```python
from build123d import *

# Parameters (mm, degrees)
MODEL_R             = 1.4605
MODEL_R_2           = 2
BOSS_EXTRUDE1_DEPTH = 2.413
SKETCH1_W           = 10
SKETCH1_H           = 24
CUT_EXTRUDE1_DEPTH  = 10


with BuildPart() as part:
    # Model → Boss-Extrude1 (new body, symmetric)
    with BuildSketch(Plane.XY):
        with BuildLine():
            Line((-290.681304326, -31.2683), (-258.931304326, -12.937428953))
            Line((-258.931304326, -12.937428953), (-258.931304326, -5.149171047))
            Line((-258.931304326, -5.149171047), (-290.681304326, 13.1817))
            Line((-290.681304326, 13.1817), (-290.681304326, 51.2817))
            Line((-290.681304326, 51.2817), (-258.931304326, 69.612571047))
            Line((-258.931304326, 69.612571047), (-258.931304326, 76.6817))
            Line((-258.931304326, 76.6817), (-290.681304326, 108.4317))
            Line((-290.681304326, 108.4317), (-290.681304326, 127.4817))
            ThreePointArc((-290.681304326, 127.4817), (-288.821432386, 131.971828061), (-284.331304326, 133.8317))
            Line((-284.331304326, 133.8317), (-265.281304326, 133.8317))
            Line((-265.281304326, 133.8317), (-227.181304326, 95.7317))
            Line((-227.181304326, 95.7317), (-23.981304326, 95.7317))
            Line((-23.981304326, 95.7317), (14.118695674, 133.8317))
            Line((14.118695674, 133.8317), (33.168695674, 133.8317))
            ThreePointArc((33.168695674, 133.8317), (37.658823735, 131.971828061), (39.518695674, 127.4817))
            Line((39.518695674, 127.4817), (39.518695674, 108.4317))
            Line((39.518695674, 108.4317), (7.768695674, 76.6817))
            Line((7.768695674, 76.6817), (7.768695674, 69.612571047))
            Line((7.768695674, 69.612571047), (39.518695674, 51.2817))
            Line((39.518695674, 51.2817), (39.518695674, 13.1817))
            Line((39.518695674, 13.1817), (7.768695674, -5.149171047))
            Line((7.768695674, -5.149171047), (7.768695674, -12.937428953))
            Line((7.768695674, -12.937428953), (39.518695674, -31.2683))
            Line((39.518695674, -31.2683), (39.518695674, -59.836710662))
            Line((39.518695674, -59.836710662), (10.464640386, -80.18057919))
            Line((10.464640386, -80.18057919), (7.768695674, -82.0683))
            Line((7.768695674, -82.0683), (7.768695674, -139.2183))
            Line((7.768695674, -139.2183), (39.518695674, -170.9683))
            Line((39.518695674, -170.9683), (39.518695674, -190.0183))
            ThreePointArc((39.518695674, -190.0183), (37.658823735, -194.508428061), (33.168695674, -196.3683))
            Line((33.168695674, -196.3683), (14.118695674, -196.3683))
            Line((14.118695674, -196.3683), (-23.981304326, -158.2683))
            Line((-23.981304326, -158.2683), (-227.181304326, -158.2683))
            Line((-227.181304326, -158.2683), (-265.281304326, -196.3683))
            Line((-265.281304326, -196.3683), (-284.331304326, -196.3683))
            ThreePointArc((-284.331304326, -196.3683), (-288.821432386, -194.508428061), (-290.681304326, -190.0183))
            Line((-290.681304326, -190.0183), (-290.681304326, -170.9683))
            Line((-290.681304326, -170.9683), (-258.931304326, -139.2183))
            Line((-258.931304326, -139.2183), (-258.931304326, -82.0683))
            Line((-258.931304326, -82.0683), (-290.681304326, -50.3183))
            Line((-290.681304326, -50.3183), (-290.681304326, -31.2683))
        make_face()
        with Locations((-287.125304326, -190.6025)):
            Circle(MODEL_R, mode=Mode.SUBTRACT)
        with Locations((33.752895674, -190.6025)):
            Circle(MODEL_R, mode=Mode.SUBTRACT)
        with Locations((33.752895674, 130.2757)):
            Circle(MODEL_R, mode=Mode.SUBTRACT)
        with Locations((-287.125304326, 130.2757)):
            Circle(MODEL_R, mode=Mode.SUBTRACT)
        with Locations((-274.681304256, -45.4288)):
            Circle(MODEL_R, mode=Mode.SUBTRACT)
        with Locations((-254.681304256, -45.4288)):
            Circle(MODEL_R, mode=Mode.SUBTRACT)
        with Locations((23.518695604, -45.4288)):
            Circle(MODEL_R, mode=Mode.SUBTRACT)
        with Locations((3.518695604, -45.4288)):
            Circle(MODEL_R, mode=Mode.SUBTRACT)
        with Locations((23.518695604, 30.5682)):
            Circle(MODEL_R, mode=Mode.SUBTRACT)
        with Locations((3.518695604, 30.5682)):
            Circle(MODEL_R, mode=Mode.SUBTRACT)
        with Locations((-254.681304256, 30.5682)):
            Circle(MODEL_R, mode=Mode.SUBTRACT)
        with Locations((-274.681304256, 30.5682)):
            Circle(MODEL_R, mode=Mode.SUBTRACT)
        with Locations((-125.581304326, -12.2183)):
            Circle(MODEL_R_2, mode=Mode.SUBTRACT)
        with Locations((-125.581304326, -50.3183)):
            Circle(MODEL_R_2, mode=Mode.SUBTRACT)
        Polygon((-30.331304326, -145.5683), (-68.431304326, -107.4683), (-182.731304326, -107.4683), (-220.831304326, -145.5683), align=None, mode=Mode.SUBTRACT)
        Polygon((-220.831304326, 83.0317), (-182.731304326, 44.9317), (-68.431304326, 44.9317), (-30.331304326, 83.0317), align=None, mode=Mode.SUBTRACT)
        Polygon((-201.781304326, -69.3683), (-233.531304326, -37.6183), (-233.531304326, -24.9183), (-201.781304326, 6.8317), (-182.731304326, 6.8317), (-150.981304326, -24.9183), (-150.981304326, -37.6183), (-182.731304326, -69.3683), align=None, mode=Mode.SUBTRACT)
        Polygon((-100.181304326, -37.6183), (-100.181304326, -24.9183), (-68.431304326, 6.8317), (-49.381304326, 6.8317), (-17.631304326, -24.9183), (-17.631304326, -37.6183), (-49.381304326, -69.3683), (-68.431304326, -69.3683), align=None, mode=Mode.SUBTRACT)
    extrude(amount=BOSS_EXTRUDE1_DEPTH, both=True)

    # Sketch1 → Cut-Extrude1 (cut)
    with BuildSketch(Plane.XY.offset(2.413)):
        with Locations((-264.681304256, -45.4288)):
            Rectangle(SKETCH1_W, SKETCH1_H)
        with Locations((-264.681304256, 30.5712)):
            Rectangle(SKETCH1_W, SKETCH1_H)
        with Locations((13.518695604, 30.5712)):
            Rectangle(SKETCH1_W, SKETCH1_H)
        with Locations((13.518695604, -45.4288)):
            Rectangle(SKETCH1_W, SKETCH1_H)
    extrude(amount=-CUT_EXTRUDE1_DEPTH, mode=Mode.SUBTRACT)


solid = part.part
```
Input: part model. Units: mm. Frame: model coordinates. A direction names the side the tool comes from. Give positions to 0.01 mm unless a question says otherwise; leave off trailing zeros. Order: outer loops, then holes, each group sorted by start corner. A loop starts at its lowest first (then second) coordinate and runs counter-clockwise, first axis right, second up. Notation, with made-up numbers: M 55.5,-38 L 94.5,-38 A25 ccw 94.5,-16 Z; hole C 4.25,35.25 d5. An arc over 180 degrees is marked long. Return JSON: item names as keys, results as strings.
Item 1: Cut plane A-A (y = 37). Return loops of the section in (x, z), then the cut area to 3 significant figures.
Solutions:
{"outline": "M -290.68,-2.41 L -269.68,-2.41 L -269.68,2.41 L -290.68,2.41 Z; M -259.68,-2.41 L 8.52,-2.41 L 8.52,2.41 L -259.68,2.41 Z; M 18.52,-2.41 L 39.52,-2.41 L 39.52,2.41 L 18.52,2.41 Z", "area": "1,500 mm^2"}
Item 2: Cut plane C-C (z = -0.4). State how many separate pieces and enclosed holes the cut face has, then the cut area to 3 significant figures.
Solutions:
{"separate pieces": "1", "enclosed holes": "22", "area": "60,200 mm^2"}
Item 3: Access query for faces 4 (the flat face through (23.866, 4.145, 0.034)), 5 (the flat face through (-167.1, -8.8, 0)), 6 (the flat face through (-275.03, 60.32, 0.03)). Directions: +Z, -Z, +X, -X, +Y, -Y. A direction counts if a zero-diameter tool reaches every point of the face in a straight line with its end or side. Return the directions, or none.
Solutions:
{"face 4": "+Z, -Z, +X", "face 5": "+Z, -Z", "face 6": "+Z, -Z, -X"}
Item 4: Pull-direction query (X, two-part tool) for faces 1 (the flat face through (23.866, 92.779, 0.034)), 2 (the flat face through (-4.665, -177.585, 0.034)), 3 (the flat face through (-275.03, -22.23, 0.03)); classes: +X half, -X half, draft (parallel to the pull), parting line (faces both ways), or undercut.
Solutions:
{"face 1": "+X half", "face 2": "undercut", "face 3": "-X half"}
Item 5: First-contact query: P1, Ø1, axis at x = 5, z = 1.5, coming from the +Y side; P2, Ø1, axis at x = -132.5, z = -1, coming from the -Y side. Flat tips, straight axial feed; report the tip coordinate or a pass-through.
Solutions:
{"P1": "y = 125.21", "P2": "y = -158.27"}
Item 6: Ray query, probe 1 along Y at (x, z) = (-138, -0.7); probe 2 along X at (y, z) = (35, -0.55); probe 3 along X at (y, z) = (-22.5, 1.1). Return the intervals inside material, ascending.
Solutions:
{"probe 1": "-158.27 to -145.57, -107.47 to 44.93, 83.03 to 95.73", "probe 2": "-290.68 to -269.68, -259.68 to 8.52, 18.52 to 39.52", "probe 3": "-275.49 to -231.11, -153.4 to -97.76, -20.05 to 24.33"}
Item 7: Cut plane B-B (x = -159). Return loops of the section in (y, z).
Solutions:
{"outline": "M -158.27,-2.41 L -145.57,-2.41 L -145.57,2.41 L -158.27,2.41 Z; M -107.47,-2.41 L -45.64,-2.41 L -45.64,2.41 L -107.47,2.41 Z; M -16.9,-2.41 L 44.93,-2.41 L 44.93,2.41 L -16.9,2.41 Z; M 83.03,-2.41 L 95.73,-2.41 L 95.73,2.41 L 83.03,2.41 Z"}
Item 8: Cut plane D-D (y = -93). Return loops of the section in (x, z), then the cut area to 3 significant figures.
Solutions:
{"outline": "M -258.93,-2.41 L 7.77,-2.41 L 7.77,2.41 L -258.93,2.41 Z", "area": "1,290 mm^2"}
